```python
from build123d import *

# Parameters (mm, degrees)
BOSS_EXTRUDE1_DEPTH = 26
FILLET1_R           = 13
CUT_EXTRUDE1_REACH  = 53.049
SKETCH2_R           = 1.5


with BuildPart() as part:
    # Sketch1 → Boss-Extrude1 (new body)
    with BuildSketch(Plane.XY):
        Polygon((0, 0), (3, 0), (3, 33), (-29, 33), (-29, 30), (0, 30), align=None)
    extrude(amount=BOSS_EXTRUDE1_DEPTH)

    # Fillet1
    fillet1_edges = [part.edges().sort_by_distance(p)[0] for p in [
        (1.5, 0, 0),
        (1.5, 0, 26),
    ]]
    fillet(fillet1_edges, radius=FILLET1_R - 0.0001)  # a hair under: the kernel refuses the full size

    # Sketch2 → Cut-Extrude1 (cut, up to next)
    with BuildSketch(Plane(origin=(0, 33, 0), x_dir=(1, 0, 0), z_dir=(0, 1, 0)), mode=Mode.PRIVATE) as cut_extrude1_sk1:
        with Locations(Location((-19.5, -5.5, 0), (0, 0, 270))):
            Circle(SKETCH2_R)
    cut_extrude1_tool1 = extrude(cut_extrude1_sk1.sketch, amount=-CUT_EXTRUDE1_REACH, mode=Mode.PRIVATE) & part.part
    # Sketch2 → Cut-Extrude1 (cut, up to next)
    with BuildSketch(Plane(origin=(0, 33, 0), x_dir=(1, 0, 0), z_dir=(0, 1, 0)), mode=Mode.PRIVATE) as cut_extrude1_sk2:
        with Locations(Location((-19.5, -20.5, 0), (0, 0, 270))):
            Circle(SKETCH2_R)
    cut_extrude1_tool2 = extrude(cut_extrude1_sk2.sketch, amount=-CUT_EXTRUDE1_REACH, mode=Mode.PRIVATE) & part.part
    # Sketch2 → Cut-Extrude1 (cut, up to next)
    with BuildSketch(Plane(origin=(0, 33, 0), x_dir=(1, 0, 0), z_dir=(0, 1, 0)), mode=Mode.PRIVATE) as cut_extrude1_sk3:
        with Locations(Location((-6.5, -5.5, 0), (0, 0, 270))):
            Circle(SKETCH2_R)
    cut_extrude1_tool3 = extrude(cut_extrude1_sk3.sketch, amount=-CUT_EXTRUDE1_REACH, mode=Mode.PRIVATE) & part.part
    # Sketch2 → Cut-Extrude1 (cut, up to next)
    with BuildSketch(Plane(origin=(0, 33, 0), x_dir=(1, 0, 0), z_dir=(0, 1, 0)), mode=Mode.PRIVATE) as cut_extrude1_sk4:
        with Locations(Location((-6.5, -20.5, 0), (0, 0, 270))):
            Circle(SKETCH2_R)
    cut_extrude1_tool4 = extrude(cut_extrude1_sk4.sketch, amount=-CUT_EXTRUDE1_REACH, mode=Mode.PRIVATE) & part.part
    add(cut_extrude1_tool1.solids().sort_by_distance((-19.5, 33, 5.5))[0], mode=Mode.SUBTRACT)
    add(cut_extrude1_tool2.solids().sort_by_distance((-19.5, 33, 20.5))[0], mode=Mode.SUBTRACT)
    add(cut_extrude1_tool3.solids().sort_by_distance((-6.5, 33, 5.5))[0], mode=Mode.SUBTRACT)
    add(cut_extrude1_tool4.solids().sort_by_distance((-6.5, 33, 20.5))[0], mode=Mode.SUBTRACT)


solid = part.part
```
The model under review builds one solid part; all positions refer to its coordinate system, in mm. A direction names the side the tool comes from. Coordinates: 2 decimals unless noted, no trailing zeros. Write each loop counter-clockwise with the first axis right and the second up, starting at its lowest first coordinate (ties: lowest second). Pieces come first, ordered by that corner, then holes. Notation, with made-up numbers: (55.5, 64) - (97.5, 64) arc R12 ccw to (97.5, 69) - close; hole circle Ø1 at (57, 88). An arc over 180 degrees is marked (long way). Answer in a Markdown table with one row per item. Add a question column.
Q1. To check wall thickness, follow line 1 along X through (y, z) = (31.2, 20.5); line 2 along Y through (x, z) = (-5, 24.75); line 3 along X through (y, z) = (18, 16.25). State the ranges of each line that lie inside material, in increasing order. Write a range as from..to.
Q2. For faces 1 (the face through (0, 15, 13)), 2 (the face through (-7.964, 31.521, 5.175)), list the 3-axis set-ups (+Z, -Z, +X, -X, +Y, -Y) from which the entire face can be reached by the end or side of a thin tool; tool diameter is ignored.
Q3. Draft analysis for pull direction Z (two halves, no side actions). For faces 3 (the face through (3, 16, 13)), 4 (the face through (1.521, 3.707, 22.091)), 5 (the face through (-18.013, 31.521, 5.305)), state which applies: +Z half, -Z half, draft (parallel to the pull), parting line (faces both ways), or undercut.
Q4. Consider section D-D on z = 12.5. Give the boundary of the cut face in (x, y).
Q5. Clearance check with flat-ended pins moving along their axes: pin 1 (13 mm diameter, centred on y = 19, z = 8.5, fed in from -X); pin 2 (3.5 mm diameter, centred on x = -19.5, z = 5.5, fed in from -Y). State where each tip first meets the part, or that it passes through.
Q6. Consider section A-A on x = -6.5. Give the boundary of the cut face in (y, z).
Q7. Consider section C-C on y = 28. Give the boundary of the cut face in (x, z).
Q8. Consider section B-B on z = 21.5. Give the boundary of the cut face in (x, y), then the cut area to 3 significant figures.
Answers below:
| question | item | result |
|---|---|---|
| 1 | line 1 | -29..-21, -18..-8, -5..3 |
| 1 | line 2 | 30..33 |
| 1 | line 3 | 0..3 |
| 2 | face 1 | +Z, -Z, -X, -Y |
| 2 | face 2 | +Y, -Y |
| 3 | face 3 | draft |
| 3 | face 4 | +Z half |
| 3 | face 5 | undercut |
| 4 | outline | (-29, 30) - (0, 30) - (0, 0.01) - (3, 0.01) - (3, 33) - (-29, 33) - close |
| 5 | pin 1 | x = 0 |
| 5 | pin 2 | y = 30 |
| 6 | outline | (30, 0) - (33, 0) - (33, 4) - (30, 4) - close; (30, 7) - (33, 7) - (33, 19) - (30, 19) - close; (30, 22) - (33, 22) - (33, 26) - (30, 26) - close |
| 7 | outline | (0, 0) - (3, 0) - (3, 26) - (0, 26) - close |
| 8 | outline | (-29, 30) - (-20.62, 30) - (-20.62, 33) - (-29, 33) - close; (-18.38, 30) - (-7.62, 30) - (-7.62, 33) - (-18.38, 33) - close; (-5.38, 30) - (0, 30) - (0, 3.16) - (3, 3.16) - (3, 33) - (-5.38, 33) - close |
| 8 | area | 163 mm² |
